Geometry check sheet. Reference: the model listing, model coordinates, mm. A direction names the side the tool comes from. Round coordinates to 2 decimals unless told otherwise and drop trailing zeros. Write each loop counter-clockwise with the first axis right and the second up, starting at its lowest first coordinate (ties: lowest second). Pieces come first, ordered by that corner, then holes.
Item 1: Scan lines: probe 1 along Z at (x, y) = (15.5, 12.5) (3 decimals); probe 2 along Z at (x, y) = (60.5, 5.5); probe 3 along Y at (x, z) = (81.5, 57.5). Record each from-to range of solid material in increasing order.
Item 2: Cross-section at C-C (y = -21). Enter the section's corners in (x, z) (3 decimals).
Item 3: Cross-section at A-A (y = -52). Enter the section's corners in (x, z) (3 decimals), then the cut area to 3 significant figures.
Item 4: Access from +Z, -Z, +X, -X, +Y, -Y to the whole of each face (thin tool, end or side, straight path). Record for faces 1 (the face through (22.225, -17, 18)), 2 (the face through (22.225, 17, 18)), 3 (the face through (59, -25.4, 45)), 4 (the face through (65, 0, 42.875)).
Item 5: Draft check along X on faces 5 (the face through (72.307, 0, 64)), 6 (the face through (98, 0, 38.1)), 7 (the face through (72.307, 0, 40)). Enter one of: pulls with the +X half, pulls with the -X half, needs draft (parallel to the pull), parting line crosses it, or undercut.
Item 6: Cross-section at B-B (x = 76.5). Enter the section's corners in (y, z) (3 decimals), then the cut area to 3 significant figures.
Item 7: Depth check by flat-ended pin: P1, Ø6, axis at x = 15.5, z = 35, coming from the +Y side; P2, Ø14, axis at y = -16, z = 19.5, coming from the -X side (3 decimals); P3, Ø6, axis at y = 8.5, z = 56.5, coming from the +X side; P4, Ø14, axis at y = 19.5, z = 15, coming from the -X side (3 decimals). Enter the tip coordinate at first touch or a pass-through.
from build123d import *

# Parameters (mm, degrees)
F1_DEPTH = 63.5
F0_W     = 25.4
F0_H     = 19.05
F0_H_2   = 4.7498
F0_H_3   = 4.7752
F2_DEPTH = 25.4
F3_DEPTH = 7.9375
F5_R     = 6.35


with BuildPart() as f1:
    # F0 (on Front) → F1 (new body, symmetric)
    with BuildSketch(Plane.XZ):
        Polygon((41.275, -9.525), (41.275, 9.525), (22.225, 9.525), (-41.275, 9.525), (-41.275, -9.525), align=None)
    extrude(amount=F1_DEPTH, both=True)

    # F0 (on Front) → F2 (join, symmetric)
    with BuildSketch(Plane.XZ):
        with BuildLine():
            Line((22.225, 9.525), (41.275, 9.525))
            Line((41.275, 9.525), (41.275, 27.0002))
            ThreePointArc((41.275, 27.0002), (45.9246798487, 38.2255201513), (57.15, 42.8752))
            Line((57.15, 42.8752), (72.3065137863, 42.8752))
            Line((72.3065137863, 42.8752), (72.3065137863, 61.9252))
            Line((72.3065137863, 61.9252), (57.15, 61.9252))
            ThreePointArc((57.15, 61.9252), (32.4542956671, 51.6959043329), (22.225, 27.0002))
            Line((22.225, 27.0002), (22.225, 9.525))
        make_face()
        with Locations((85.0065137863, 52.4002)):
            Rectangle(F0_W, F0_H)
        with Locations((85.0065137863, 64.3001)):
            Rectangle(F0_W, F0_H_2)
        with Locations((85.0065137863, 40.4876)):
            Rectangle(F0_W, F0_H_3)
    extrude(amount=F2_DEPTH, both=True)

    # F0 (on Front) → F3 (join, symmetric)
    with BuildSketch(Plane.XZ):
        with BuildLine():
            Line((-41.275, 9.525), (22.225, 9.525))
            Line((22.225, 9.525), (22.225, 27.0002))
            ThreePointArc((22.225, 27.0002), (32.4542956671, 51.6959043329), (57.15, 61.9252))
            add(Edge.make_bspline(
                [(-41.275, 9.525), (-29.7216698527, 55.1520250738), (24.5722677241, 62.3028567907), (57.15, 61.9252)],
                knots=[0, 0, 0, 0, 111.5045361635, 111.5045361635, 111.5045361635, 111.5045361635], degree=3))
        make_face()
    extrude(amount=F3_DEPTH, both=True)

    # F0 (on Front) → F4 (revolve)
    with BuildSketch(Plane.XZ):
        Polygon((97.7065137863, 61.9252), (97.7065137863, 42.8752), (97.7065137863, 38.1), (123.1065137863, 38.1), (123.1065137863, 66.675), (97.7065137863, 66.675), align=None)
    revolve(axis=Axis((97.7065137863, 0, 52.3875), (0, 0, 1)))

    # F5
    f5_edges = [f1.edges().sort_by_distance(p)[0] for p in [
        (41.275, -63.5, 0),
        (41.275, 63.5, 0),
        (-41.275, 63.5, 0),
        (-41.275, -63.5, 0),
    ]]
    fillet(f5_edges, radius=F5_R)


solid = f1.part
Resolved:
1. probe 1: z = -9.525 to 9.525
1. probe 2: z = 42.88 to 61.93
1. probe 3: y = -25.4 to 25.4
2. outline: (-41.275, -9.525) - (41.275, -9.525) - (41.275, 27) arc R15.875 cw to (57.15, 42.875) - (72.307, 42.875) - (72.307, 38.1) - (111.995, 38.1) - (111.995, 66.675) - (72.307, 66.675) - (72.307, 61.925) - (57.15, 61.925) arc R34.925 ccw to (22.225, 27) - (22.225, 9.525) - (-41.275, 9.525) - close
3. outline: (-41.275, -9.525) - (41.275, -9.525) - (41.275, 9.525) - (-41.275, 9.525) - close
3. area: 1,570 mm2
4. face 1: +Z, -X, -Y
4. face 2: +Z, -X, +Y
4. face 3: +Z, +X, -X, -Y
4. face 4: -Z, +Y, -Y
5. face 5: pulls with the -X half
5. face 6: needs draft
5. face 7: undercut
6. outline: (-25.4, 38.1) - (25.4, 38.1) - (25.4, 66.675) - (-25.4, 66.675) - close
6. area: 1,450 mm2
7. P1: stops at y = 7.94
7. P2: stops at x = 22.225
7. P3: stops at x = 122.5
7. P4: stops at x = -41.275
